Input: dimensioned drawing with shaded views. Units: mm. Origin: part minimum x, y, z. Round coordinates to 2 decimals unless told otherwise and drop trailing zeros. Write each loop counter-clockwise with the first axis right and the second up, starting at its lowest first coordinate (ties: lowest second). Pieces come first, ordered by that corner, then holes. Notation, with made-up numbers: M -18,58 L -3,58 A23 ccw -3,67 Z; hole C 25,-2 d8. An arc over 180 degrees is marked long. Answer in a Markdown table with one row per item. Add a question column.
Item 1: Cut plane C-C on z = 59.5. Return loops of the section in (x, y).
Item 2: Contact query for flat-ended pins moving along their axis: pin 1 (5 mm diameter, centred on y = 20.5, z = 23.5, fed in from -X); pin 2 (3.5 mm diameter, centred on x = 12.7, y = 12.7, fed in from +Z); pin 3 (2 mm diameter, centred on y = 15, z = 73.5, fed in from -X); pin 4 (12 mm diameter, centred on y = 21, z = 18, fed in from -X). Output: stop coordinate, or through.
Item 3: Cut plane A-A on x = 12.7. Return loops of the section in (y, z), and give its area (3 significant figures).
Item 4: Material intervals for probe 1 along Y at (x, z) = (12.7, 66); probe 2 along Y at (x, z) = (12, 35.5) (1 decimal); probe 3 along Y at (x, z) = (4.5, 60), sorted ascending.
Item 5: Cut plane D-D on y = 17. Return loops of the section in (x, z), and give its area (3 significant figures).
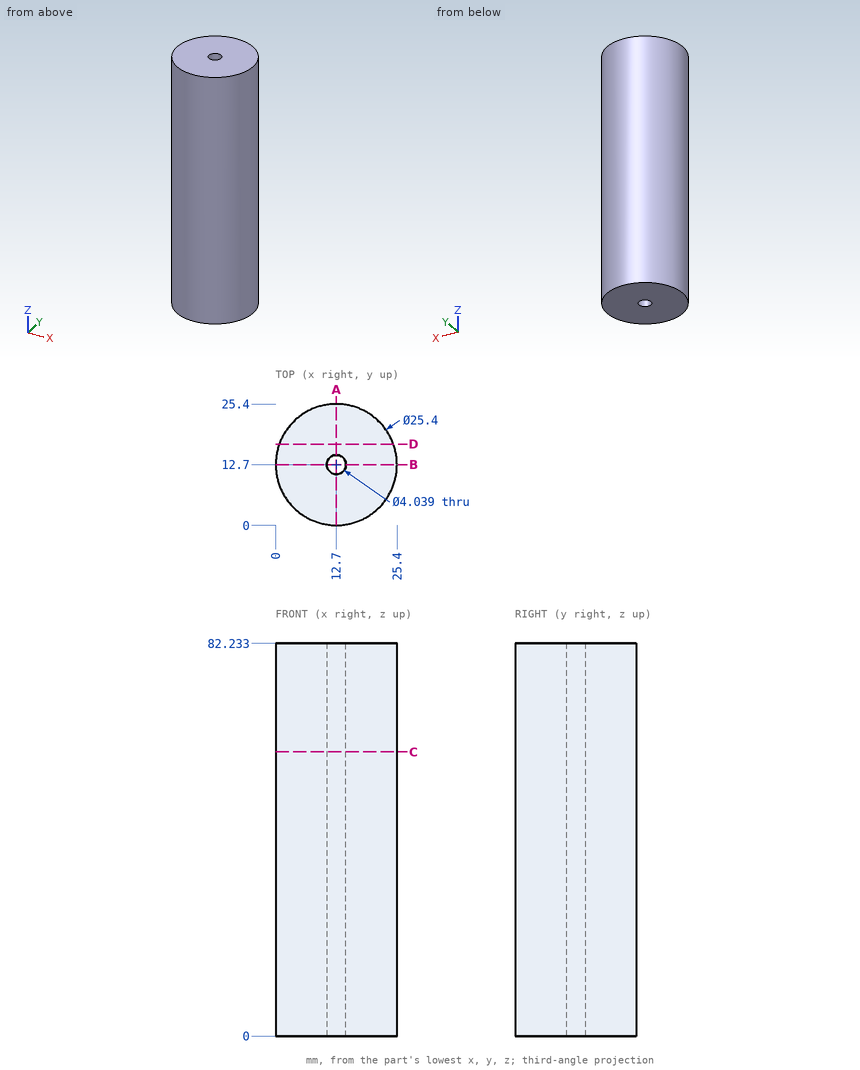
Results below:
| question | item | result |
|---|---|---|
| 1 | outline | C 12.7,12.7 d25.4; hole C 12.7,12.7 d4.04 |
| 2 | pin 1 | x = 1.16 |
| 2 | pin 2 | through |
| 2 | pin 3 | x = 0.07 |
| 2 | pin 4 | x = 0.21 |
| 3 | outline | M 0,0 L 10.68,0 L 10.68,82.23 L 0,82.23 Z; M 14.72,0 L 25.4,0 L 25.4,82.23 L 14.72,82.23 Z |
| 3 | area | 1,760 mm2 |
| 4 | probe 1 | 0 to 10.68, 14.72 to 25.4 |
| 4 | probe 2 | 0 to 10.8, 14.6 to 25.4 |
| 4 | probe 3 | 3 to 22.4 |
| 5 | outline | M 0.75,0 L 24.65,0 L 24.65,82.23 L 0.75,82.23 Z |
| 5 | area | 1,970 mm2 |
